Read the model definition and answer for the solid it produces. Units are mm, in the model's axes. A direction names the side the tool comes from. Coordinates: 2 decimals unless noted, no trailing zeros. Order: outer loops, then holes, each group sorted by start corner. A loop starts at its lowest first (then second) coordinate and runs counter-clockwise, first axis right, second up. Notation, with made-up numbers: (-29, 0.25) -> (21, 0.25) arc R29 ccw to (21, 32.25) -> close; hole circle Ø5 at (-36.75, 23). An arc over 180 degrees is marked (long way). Answer in a Markdown table with one row per item.
from build123d import *

# Parameters (mm, degrees)
F1_DEPTH = 2.5
F2_R     = 0.85
F3_DEPTH = 12.5


with BuildPart() as f1:
    # F0 (on Top) → F1 (new body)
    with BuildSketch(Plane.XY):
        with BuildLine():
            Line((13.081475452, -13.081475452), (1.0606601718, -1.0606601718))
            ThreePointArc((1.0606601718, -1.0606601718), (0, -0.6213203436), (-1.0606601718, -1.0606601718))
            Line((-1.0606601718, -1.0606601718), (-13.081475452, -13.081475452))
            ThreePointArc((-13.081475452, -13.081475452), (-13.5208152802, -14.1421356237), (-13.081475452, -15.2027957955))
            Line((-13.081475452, -15.2027957955), (-1.0606601718, -27.2236110757))
            ThreePointArc((-1.0606601718, -27.2236110757), (0, -27.6629509039), (1.0606601718, -27.2236110757))
            Line((1.0606601718, -27.2236110757), (13.081475452, -15.2027957955))
            ThreePointArc((13.081475452, -15.2027957955), (13.5208152802, -14.1421356237), (13.081475452, -13.081475452))
        make_face()
        with BuildLine():
            Line((-2.3015444974, -7.3716045666), (-2.3015444974, -12.3292868583))
            Line((-2.3015444974, -12.3292868583), (-2.9590965807, -12.3292868583))
            Line((-2.9590965807, -12.3292868583), (-5.6685149835, -8.1691306083))
            Line((-5.6685149835, -8.1691306083), (-5.6956417196, -8.1691306083))
            add(Edge.make_bspline(
                [(-5.6956417196, -8.1691306083), (-5.6413882474, -8.9015524833), (-5.6413882474, -9.5113615111)],
                knots=[0, 0, 0, 1, 1, 1], degree=2))
            Line((-5.6413882474, -9.5113615111), (-5.6413882474, -12.3292868583))
            Line((-5.6413882474, -12.3292868583), (-6.1741573446, -12.3292868583))
            Line((-6.1741573446, -12.3292868583), (-6.1741573446, -7.3716045666))
            Line((-6.1741573446, -7.3716045666), (-5.523115678, -7.3716045666))
            Line((-5.523115678, -7.3716045666), (-2.8202076919, -11.515484775))
            Line((-2.8202076919, -11.515484775), (-2.7930809557, -11.515484775))
            add(Edge.make_bspline(
                [(-2.7930809557, -11.515484775), (-2.7995913724, -11.4243389416), (-2.8234629002, -10.9273771361)],
                knots=[0, 0, 0, 1, 1, 1], degree=2))
            add(Edge.make_bspline(
                [(-2.8234629002, -10.9273771361), (-2.847334428, -10.4304153305), (-2.8408240113, -10.21665665)],
                knots=[0, 0, 0, 1, 1, 1], degree=2))
            Line((-2.8408240113, -10.21665665), (-2.8408240113, -7.3716045666))
            Line((-2.8408240113, -7.3716045666), (-2.3015444974, -7.3716045666))
        make_face(mode=Mode.SUBTRACT)
        with BuildLine():
            Line((-8.1334756687, -14.8039748892), (-8.1334756687, -13.4802963582))
            Line((-8.1334756687, -13.4802963582), (-0.6236797201, -13.4802963582))
            Line((-0.6236797201, -13.4802963582), (-0.6236797201, -6.9198086858))
            ThreePointArc((-0.6236797201, -6.9198086858), (-0.9032194318, -6.4583786209), (-0.9135835525, -5.9189782686))
            ThreePointArc((-0.9135835525, -5.9189782686), (0.0168397474, -5.0141534426), (0.9868078824, -5.876451129))
            ThreePointArc((0.9868078824, -5.876451129), (0.9900106564, -6.4384308628), (0.6999988109, -6.9198086858))
            Line((0.6999988109, -6.9198086858), (0.6999988109, -13.4802963582))
            Line((0.6999988109, -13.4802963582), (8.1334756687, -13.4802963582))
            ThreePointArc((8.1334756687, -13.4802963582), (8.5949057336, -13.2007566465), (9.134306086, -13.1903925258))
            ThreePointArc((9.134306086, -13.1903925258), (10.0391309119, -14.1208158258), (9.1768332255, -15.0907839607))
            ThreePointArc((9.1768332255, -15.0907839607), (8.6148534917, -15.0939867347), (8.1334756687, -14.8039748892))
            Line((8.1334756687, -14.8039748892), (0.6999988109, -14.8039748892))
            Line((0.6999988109, -14.8039748892), (0.6999988109, -23.1867600232))
            Line((0.6999988109, -23.1867600232), (-0.6236797201, -23.1867600232))
            Line((-0.6236797201, -23.1867600232), (-0.6236797201, -14.8039748892))
            Line((-0.6236797201, -14.8039748892), (-8.1334756687, -14.8039748892))
        make_face(mode=Mode.SUBTRACT)
        with BuildLine():
            add(Edge.make_bspline(
                [(5.5299358711, -10.0878473268), (5.8229046211, -10.4068577434), (5.8229046211, -10.9146702434)],
                knots=[0, 0, 0, 1, 1, 1], degree=2))
            add(Edge.make_bspline(
                [(5.8229046211, -10.9146702434), (5.8229046211, -11.5689671184), (5.3481867392, -11.9357205907)],
                knots=[0, 0, 0, 1, 1, 1], degree=2))
            add(Edge.make_bspline(
                [(5.3481867392, -11.9357205907), (4.8734688573, -12.3024740629), (4.0596667739, -12.3024740629)],
                knots=[0, 0, 0, 1, 1, 1], degree=2))
            add(Edge.make_bspline(
                [(4.0596667739, -12.3024740629), (3.178590385, -12.3024740629), (2.7033299684, -12.0746094796)],
                knots=[0, 0, 0, 1, 1, 1], degree=2))
            Line((2.7033299684, -12.0746094796), (2.7033299684, -11.519053924))
            add(Edge.make_bspline(
                [(2.7033299684, -11.519053924), (3.0093195517, -11.6470921184), (3.3684775378, -11.7219619101)],
                knots=[0, 0, 0, 1, 1, 1], degree=2))
            add(Edge.make_bspline(
                [(3.3684775378, -11.7219619101), (3.7276355239, -11.7968317018), (4.0802830934, -11.7968317018)],
                knots=[0, 0, 0, 1, 1, 1], degree=2))
            add(Edge.make_bspline(
                [(4.0802830934, -11.7968317018), (4.6564549684, -11.7968317018), (4.9483386489, -11.5781902087)],
                knots=[0, 0, 0, 1, 1, 1], degree=2))
            add(Edge.make_bspline(
                [(4.9483386489, -11.5781902087), (5.2402223295, -11.3595487157), (5.2402223295, -10.9689237157)],
                knots=[0, 0, 0, 1, 1, 1], degree=2))
            add(Edge.make_bspline(
                [(5.2402223295, -10.9689237157), (5.2402223295, -10.7117622573), (5.1365981975, -10.5473742365)],
                knots=[0, 0, 0, 1, 1, 1], degree=2))
            add(Edge.make_bspline(
                [(5.1365981975, -10.5473742365), (5.0329740656, -10.3829862157), (4.7904610448, -10.2435547921)],
                knots=[0, 0, 0, 1, 1, 1], degree=2))
            add(Edge.make_bspline(
                [(4.7904610448, -10.2435547921), (4.5479480239, -10.1041233684), (4.0531563573, -9.9283421184)],
                knots=[0, 0, 0, 1, 1, 1], degree=2))
            add(Edge.make_bspline(
                [(4.0531563573, -9.9283421184), (3.3619671211, -9.6809462851), (3.0652006281, -9.3418620837)],
                knots=[0, 0, 0, 1, 1, 1], degree=2))
            add(Edge.make_bspline(
                [(3.0652006281, -9.3418620837), (2.768434135, -9.0027778823), (2.768434135, -8.4569879518)],
                knots=[0, 0, 0, 1, 1, 1], degree=2))
            add(Edge.make_bspline(
                [(2.768434135, -8.4569879518), (2.768434135, -7.8840712851), (3.1986641698, -7.5449870837)],
                knots=[0, 0, 0, 1, 1, 1], degree=2))
            add(Edge.make_bspline(
                [(3.1986641698, -7.5449870837), (3.6288942045, -7.2059028823), (4.3385296211, -7.2059028823)],
                knots=[0, 0, 0, 1, 1, 1], degree=2))
            add(Edge.make_bspline(
                [(4.3385296211, -7.2059028823), (5.0774619128, -7.2059028823), (5.698121635, -7.4771702434)],
                knots=[0, 0, 0, 1, 1, 1], degree=2))
            Line((5.698121635, -7.4771702434), (5.5180001073, -7.9784723268))
            add(Edge.make_bspline(
                [(5.5180001073, -7.9784723268), (4.9038508017, -7.7213108684), (4.3244237184, -7.7213108684)],
                knots=[0, 0, 0, 1, 1, 1], degree=2))
            add(Edge.make_bspline(
                [(4.3244237184, -7.7213108684), (3.8665244128, -7.7213108684), (3.6088204198, -7.9177084379)],
                knots=[0, 0, 0, 1, 1, 1], degree=2))
            add(Edge.make_bspline(
                [(3.6088204198, -7.9177084379), (3.3511164267, -8.1141060073), (3.3511164267, -8.4634983684)],
                knots=[0, 0, 0, 1, 1, 1], degree=2))
            add(Edge.make_bspline(
                [(3.3511164267, -8.4634983684), (3.3511164267, -8.7206598268), (3.4460600031, -8.8855903823)],
                knots=[0, 0, 0, 1, 1, 1], degree=2))
            add(Edge.make_bspline(
                [(3.4460600031, -8.8855903823), (3.5410035795, -9.0505209379), (3.7666980239, -9.1877822226)],
                knots=[0, 0, 0, 1, 1, 1], degree=2))
            add(Edge.make_bspline(
                [(3.7666980239, -9.1877822226), (3.9923924684, -9.3250435073), (4.4568021906, -9.4910591323)],
                knots=[0, 0, 0, 1, 1, 1], degree=2))
            add(Edge.make_bspline(
                [(4.4568021906, -9.4910591323), (5.2369671211, -9.7688369101), (5.5299358711, -10.0878473268)],
                knots=[0, 0, 0, 1, 1, 1], degree=2))
        make_face(mode=Mode.SUBTRACT)
    extrude(amount=F1_DEPTH)

    # F2 (on Right) → F3 (cut, symmetric)
    with BuildSketch(Plane.YZ):
        with Locations((-2.4908210296, 1.292226194)):
            Circle(F2_R)
    extrude(amount=F3_DEPTH, both=True, mode=Mode.SUBTRACT)


solid = f1.part
Q1. The part is cut by section A-A (x = 6.25). Write down the section's boundary in (y, z), then the cut area to 3 significant figures.
Outcome:
| item | result |
|---|---|
| outline | (-22.03, 0) -> (-14.8, 0) -> (-14.8, 2.5) -> (-22.03, 2.5) -> close; (-13.48, 0) -> (-6.25, 0) -> (-6.25, 2.5) -> (-13.48, 2.5) -> close |
| area | 36.2 mm² |
Q2. The part is cut by section C-C (z = 1.6). Give the number of separate pieces and of enclosed holes in the cut face, then the cut area to 3 significant figures.
Outcome:
| item | result |
|---|---|
| separate pieces | 2 |
| enclosed holes | 3 |
| area | 329 mm² |
Q3. Given pin 1 (0.5 mm diameter, centred on x = -6, z = 1.5, fed in from -Y); pin 2 (1.2 mm diameter, centred on y = -11, z = 1.5, fed in from +X), each flat-ended and moving along its own axis, determine where each tip first touches the part or whether it passes through.
Outcome:
| item | result |
|---|---|
| pin 1 | y = -22.53 |
| pin 2 | x = 11.6 |
Q4. For faces 4 (the face through (13.52, -14.16, 1.23)), 5 (the face through (4, -13.48, 1)), determine the directions among +Z, -Z, +X, -X, +Y, -Y from which every point of the face is accessible in a straight line to the end or side of a thin tool.
Outcome:
| item | result |
|---|---|
| face 4 | +Z, -Z, +X |
| face 5 | +Z, -Z |
Q5. The part is cut by section D-D (x = -4.75). Write down the section's boundary in (y, z), then the cut area to 3 significant figures.
Outcome:
| item | result |
|---|---|
| outline | (-23.53, 0) -> (-14.8, 0) -> (-14.8, 2.5) -> (-23.53, 2.5) -> close; (-13.48, 0) -> (-9.58, 0) -> (-9.58, 2.5) -> (-13.48, 2.5) -> close; (-8.56, 0) -> (-4.75, 0) -> (-4.75, 2.5) -> (-8.56, 2.5) -> close |
| area | 41.1 mm² |
Q6. The part is cut by section B-B (y = -17). Write down the section's boundary in (x, z), then the cut area to 3 significant figures.
Outcome:
| item | result |
|---|---|
| outline | (-11.28, 0) -> (-0.62, 0) -> (-0.62, 2.5) -> (-11.28, 2.5) -> close; (0.7, 0) -> (11.28, 0) -> (11.28, 2.5) -> (0.7, 2.5) -> close |
| area | 53.1 mm² |
Q7. Consider line 1 (Y direction, x = 1.5, z = 0.8); line 2 (Y direction, x = 0.75, z = 1.15); line 3 (Y direction, x = -2.75, z = 0.95). Determine where each line is inside the solid, lowest interval first.
Outcome:
| item | result |
|---|---|
| line 1 | -26.78 to -14.8, -13.48 to -3.18, -1.8 to -1.5 |
| line 2 | -27.46 to -14.8, -13.48 to -6.87, -5.33 to -3.33, -1.65 to -0.82 |
| line 3 | -25.53 to -14.8, -13.48 to -12.33, -7.37 to -3.27 |
Q8. For a pull along X with two mould halves and no side action, classify faces 1 (the face through (0.02, -0.62, 1.23)), 2 (the face through (-1, -15, 2.5)), 3 (the face through (0.7, -10, 1)) as pulls with the +X half, pulls with the -X half, needs draft (parallel to the pull), parting line crosses it, or undercut.
Outcome:
| item | result |
|---|---|
| face 1 | parting line crosses it |
| face 2 | needs draft |
| face 3 | undercut |
